CAD build for the part. Positions are in the model's coordinates, mm. Face numbers are marked on the shaded views. A direction names the side the tool comes from. Coordinates: 2 decimals unless noted, no trailing zeros. Loops run counter-clockwise (first coordinate to the right, second up) from the corner with the lowest first, then second, coordinate; pieces in that order, holes last. Notation, with made-up numbers: (47.25, 38) - (74.25, 38) arc R18 cw to (74.25, 55) - close; hole circle Ø5 at (-14, -33). An arc over 180 degrees is marked (long way). Put each result on its own line as item: value.
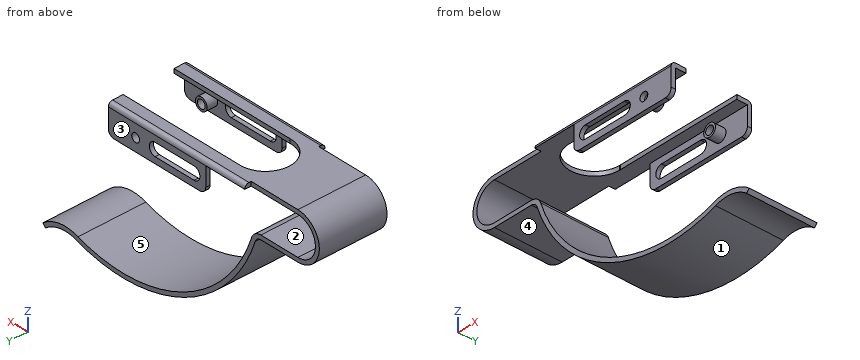
```python
from build123d import *

# Parameters (mm, degrees)
F1_DEPTH  = 16
F2_W      = 70
F2_H      = 3
F3_DEPTH  = 2
F4_W      = 50
F4_H      = 14
F5_DEPTH  = 2
F6_R      = 2
F9_DEPTH  = 2
F11_DEPTH = 38.001
F13_D     = 4
F14_R     = 3
F14_R_2   = 2
F15_DEPTH = 5
F16_R     = 3


# Not quite as in the source:
# - a pattern or mirror of a feature is missing from the dataset's text; its kind, count and spacing are read off the source's solid


with BuildPart() as f1:
    # F0 (on Front) → F1 (new body)
    with BuildSketch(Plane.XZ):
        with BuildLine():
            ThreePointArc((0, -9), (-9, 0), (0, 9))
            Line((0, 9), (94, 9))
            Line((94, 9), (94, 11))
            Line((94, 11), (0, 11))
            ThreePointArc((0, 11), (-11, 0), (0, -11))
            Line((0, -11), (19, -11))
            ThreePointArc((19, -11), (20.7464347921, -11.5607448848), (21.84, -13.0333563221))
            ThreePointArc((21.84, -13.0333563221), (58.3659358906, -54.5122350868), (113.5320571839, -57.8797917247))
            ThreePointArc((113.5320571839, -57.8797917247), (121.8779484376, -57.0367571838), (129.5033807995, -60.5320954149))
            Line((129.5033807995, -60.5320954149), (130.788961497, -59))
            ThreePointArc((130.788961497, -59), (122.2254958147, -55.0670941025), (112.8483757943, -56))
            ThreePointArc((112.8483757943, -56), (59.2303979034, -52.7086373708), (23.7333333333, -12.3889272035))
            ThreePointArc((23.7333333333, -12.3889272035), (21.9107246536, -9.9345748081), (19, -9))
            Line((19, -9), (0, -9))
        make_face()
    extrude(amount=F1_DEPTH)

    # F2 (on face) → F3 (join)
    with BuildSketch(Plane.XY.offset(11)):
        with Locations((59, -17.5)):
            Rectangle(F2_W, F2_H)
    extrude(amount=-F3_DEPTH)

    # F4 (on face) → F5 (join)
    with BuildSketch(Plane.XZ.offset(19)):
        with Locations((69, 4)):
            Rectangle(F4_W, F4_H)
    extrude(amount=-F5_DEPTH)

    # F6
    f6_edges = [f1.edges().sort_by_distance(p)[0] for p in [
        (59, -19, 11),
    ]]
    fillet(f6_edges, radius=F6_R)

    # F7: F1 across plane


with BuildPart() as f1_1:
    add(f1.part)
    add(f1.part.mirror(Plane.XZ))

    # F8 (on face) → F9 (cut)
    with BuildSketch(Plane.XY.offset(11)):
        with BuildLine():
            Line((33.6929396674, 11.9960707714), (34.3070603326, 11.9960707714))
            ThreePointArc((34.3070603326, 11.9960707714), (34, 12), (33.6929396674, 11.9960707714))
        make_face()
        with BuildLine():
            Line((94, 11.9960707714), (34.3070603326, 11.9960707714))
            Line((34.3070603326, 11.9960707714), (33.6929396674, 11.9960707714))
            ThreePointArc((33.6929396674, 11.9960707714), (22.0074226206, -0.4220045025), (34.5369099172, -11.9879826385))
            Line((34.5369099172, -11.9879826385), (94, -11.9879826385))
            Line((94, -11.9879826385), (94, 11.9960707714))
        make_face()
    extrude(amount=-F9_DEPTH, mode=Mode.SUBTRACT)

    # F10 (on face) → F11 (cut, through all)
    with BuildSketch(Plane.XZ.offset(19)):
        with BuildLine():
            ThreePointArc((50, 6), (47, 3), (50, 0))
            Line((50, 0), (70, 0))
            ThreePointArc((70, 0), (73, 3), (70, 6))
            Line((70, 6), (50, 6))
        make_face()
    extrude(amount=-F11_DEPTH, mode=Mode.SUBTRACT)

    # F13 (through all)
    with Locations(Plane.XZ.offset(19)):
        with Locations((80, 3)):
            Hole(F13_D / 2)

    # F14 (on face) → F15 (join)
    with BuildSketch(Plane(origin=(0, -17, 0), x_dir=(-1, 0, 0), z_dir=(0, 1, 0))):
        with Locations((-80, 3)):
            Circle(F14_R)
        with Locations((-80, 3)):
            Circle(F14_R_2, mode=Mode.SUBTRACT)
    f15 = extrude(amount=F15_DEPTH)

    # F15_copies: F15 across plane
    add(f15.mirror(Plane.ZX))

    # F16
    f16_edges = [f1_1.edges().sort_by_distance(p)[0] for p in [
        (44, 18, -3),
        (44, -18, -3),
        (94, 18, -3),
        (94, -18, -3),
    ]]
    fillet(f16_edges, radius=F16_R)


solid = f1_1.part
```
Q1. Slice it at A-A, the plane x = 86.5. Give the cut face in (y, z).
Determined:
outline: (-19, -3) - (-17, -3) - (-17, 9) - (-11.99, 9) - (-11.99, 11) - (-17, 11) arc R2 ccw to (-19, 9) - close; (-16, -61.75) - (16, -61.75) - (16, -59.75) - (-16, -59.75) - close; (12, 9) - (17, 9) - (17, -3) - (19, -3) - (19, 9) arc R2 ccw to (17, 11) - (12, 11) - close
Q2. Mould opens along Z. For the marked faces 3, 4 and 5 say: +Z half, -Z half, draft (parallel to the pull), parting line (faces both ways), or undercut.
Determined:
face 3: draft
face 4: -Z half
face 5: undercut
Q3. Slice it at D-D, the plane z = 3. State how many separate pieces and enclosed holes the cut face has, then the cut area to 3 significant figures.
Determined:
separate pieces: 7
enclosed holes: 0
area: 167 mm2
Q4. Wall check: L1, parallel to Z at x = 80, y = 14.5; L2, parallel to Z at x = 42, y = 15.5; L3, parallel to Y at x = 47, z = 2.5. Give the ranges that are in metal, low to high. Write a range as from..to.
Determined:
L1: -61.14..-59.12, 0..1, 5..6, 9..11
L2: -43.5..-40.78, 9..11
L3: -19..-17, 17..19
Q5. Slice it at C-C, the plane x = 54.5. Give the cut face in (y, z).
Determined:
outline: (-19, -3) - (-17, -3) - (-17, 0) - (-19, 0) - close; (-19, 6) - (-17, 6) - (-17, 9) - (-11.99, 9) - (-11.99, 11) - (-17, 11) arc R2 ccw to (-19, 9) - close; (-16, -52.47) - (16, -52.47) - (16, -50.16) - (-16, -50.16) - close; (12, 9) - (17, 9) - (17, 6) - (19, 6) - (19, 9) arc R2 ccw to (17, 11) - (12, 11) - close; (17, -3) - (19, -3) - (19, 0) - (17, 0) - close
Q6. Slice it at B-B, the plane y = 2. Give the cut face in (x, z).
Determined:
outline: (0, -11) - (19, -11) arc R3 cw to (21.84, -13.03) arc R72 ccw to (113.53, -57.88) arc R16 cw to (129.5, -60.53) - (130.79, -59) arc R18 ccw to (112.85, -56) arc R70 cw to (23.73, -12.39) arc R5 ccw to (19, -9) - (0, -9) arc R9 cw to (0, 9) - (22.17, 9) - (22.17, 11) - (0, 11) arc R11 ccw to start
Q7. Pin check, flat tips, straight feed: pin 1 Ø1 at (x, y) = (75, 18.5) entering from -Z; pin 2 Ø1 at (y, z) = (5, -25) entering from +X; pin 3 Ø1.6 at (y, z) = (18, 6.5) entering from -X. Stop position of each tip, or through.
Determined:
pin 1: z = -3
pin 2: x = 29.77
pin 3: x = 44
Q8. Tool access for the marked faces 1 and 2: list every direction of +Z, -Z, +X, -X, +Y, -Y with a clear straight run to the whole face (end or side of a thin tool).
Determined:
face 1: -Z, +Y, -Y
face 2: +X, +Y, -Y
